```python
from build123d import *

# Parameters (mm, degrees)
F0_W      = 19.05
F0_H      = 19.05
F1_DEPTH  = 11.43
F3_DEPTH  = 19.051
F5_DEPTH  = 19.051
F6_R      = 4.445
F6_R_2    = 1.807104104
F7_DEPTH  = 19.05
F8_DEPTH  = 19.0510001
F9_W      = 2.54
F9_H      = 19.05
F10_DEPTH = 19.0510001
F11_W     = 13.97
F11_H     = 13.97
F11_R     = 4.445
F12_DEPTH = 6.35
F13_R     = 1.27


with BuildPart() as f1:
    # F0 (on Front) → F1 (new body)
    with BuildSketch(Plane.XZ):
        Rectangle(F0_W, F0_H)
    extrude(amount=F1_DEPTH)

    # F2 (on face) → F3 (cut, through all)
    with BuildSketch(Plane.YZ.offset(9.525)):
        with BuildLine():
            Line((0, -9.525), (0, 9.525))
            ThreePointArc((0, 9.525), (-2.032, 0), (0, -9.525))
        make_face()
    extrude(amount=-F3_DEPTH, mode=Mode.SUBTRACT)

    # F4 (on face) → F5 (cut, through all)
    with BuildSketch(Plane.XY.offset(9.525)):
        with BuildLine():
            ThreePointArc((9.525, 0), (19.5841950931, 8.6107735797), (23.34021875, 21.30821875))
            ThreePointArc((23.34021875, 21.30821875), (-12.6974451703, 40.8924138431), (-9.525, 0))
            Line((-9.525, 0), (9.525, 0))
        make_face()
        with BuildLine():
            Line((9.525, 0), (-9.525, 0))
            ThreePointArc((-9.525, 0), (0, -2.032), (9.525, 0))
        make_face()
    extrude(amount=-F5_DEPTH, mode=Mode.SUBTRACT)

    # F6 (on face) → F7 (join)
    with BuildSketch(Plane.XZ.offset(11.43)):
        Circle(F6_R)
        Circle(F6_R_2, mode=Mode.SUBTRACT)
    extrude(amount=-F7_DEPTH)

    # F6 (on face) → F8 (cut, through all)
    with BuildSketch(Plane.XZ.offset(11.43)):
        Circle(F6_R_2)
    extrude(amount=-F8_DEPTH, mode=Mode.SUBTRACT)

    # F9 (on face) → F10 (cut, through all)
    with BuildSketch(Plane.YZ.offset(9.525)):
        with Locations((-10.16, 0)):
            Rectangle(F9_W, F9_H)
    extrude(amount=-F10_DEPTH, mode=Mode.SUBTRACT)

    # F11 (on face) + F6 (on face) → F12 (cut)
    with BuildSketch(Plane.XZ.offset(11.43)):
        Rectangle(F11_W, F11_H)
        Circle(F11_R, mode=Mode.SUBTRACT)
    with BuildSketch(Plane.XZ.offset(11.43)):
        Circle(F6_R)
        Circle(F6_R_2, mode=Mode.SUBTRACT)
    extrude(amount=-F12_DEPTH, mode=Mode.SUBTRACT)

    # F13
    f13_edges = [f1.edges().sort_by_distance(p)[0] for p in [
        (-9.525, -4.445, -9.525),
        (-9.525, -4.445, 9.525),
        (9.525, -4.445, 9.525),
        (9.525, -4.445, -9.525),
    ]]
    fillet(f13_edges, radius=F13_R)


solid = f1.part
```
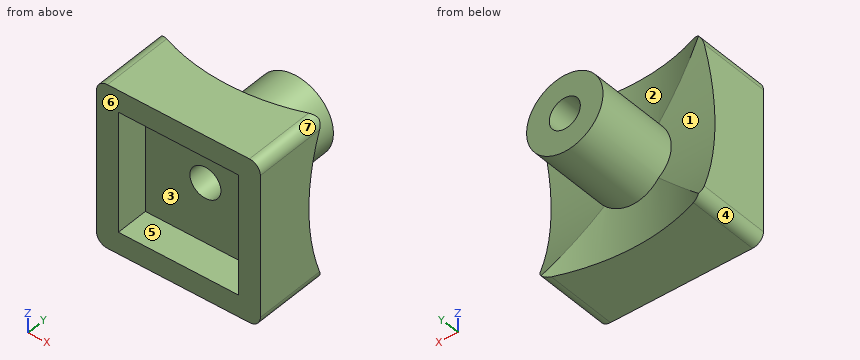
Verification items for the finished model (mm, model axes). Face numbers are marked on the shaded views. A direction names the side the tool comes from. Round coordinates to 2 decimals unless told otherwise and drop trailing zeros. Write each loop counter-clockwise with the first axis right and the second up, starting at its lowest first coordinate (ties: lowest second). Pieces come first, ordered by that corner, then holes.
1. Section check A-A on x = 0. Enter the section's corners in (y, z) (3 decimals), plus the area to 3 significant figures.
2. Gauge pin test, flat ends, axial feed: P1, Ø5, axis at x = 7.5, y = 3.5, coming from the +Z side; P2, Ø7, axis at x = 0.5, z = -3, coming from the -Y side; P3, Ø2, axis at x = -2.5, y = 2, coming from the +Z side; P4, Ø3, axis at x = 2, y = 2.5, coming from the -Z side. Record the tip position at first contact, or that the pin passes through.
3. Section check D-D on x = 5.75. Enter the section's corners in (y, z) (3 decimals), plus the area to 3 significant figures.
4. Scan lines: L1, parallel to X at y = 0.75, z = 0 (3 decimals); L2, parallel to X at y = -3.5, z = 0 (3 decimals). Record each from-to range of solid material in increasing order.
5. Draft check along X on the marked faces 4, 5, 6 and 7. Enter one of: +X half, -X half, draft (parallel to the pull), parting line (faces both ways), or undercut.
6. Section check C-C on z = 0. Enter the section's corners in (x, y) (3 decimals), plus the area to 3 significant figures.
7. Section check B-B on y = -1.25. Enter the section's corners in (x, z) (3 decimals).
8. Access from +Z, -Z, +X, -X, +Y, -Y to the whole of each face (thin tool, end or side, straight path). Record for the marked faces 1, 2 and 3.
Answer:
1. outline: (-8.89, -9.525) - (-2.032, -9.525) - (-2.032, -4.445) - (7.62, -4.445) - (7.62, -1.807) - (-5.08, -1.807) - (-5.08, -6.985) - (-8.89, -6.985) - close; (-8.89, 6.985) - (-5.08, 6.985) - (-5.08, 1.807) - (7.62, 1.807) - (7.62, 4.445) - (-2.032, 4.445) - (-2.032, 9.525) - (-8.89, 9.525) - close
1. area: 117 mm2
2. P1: passes through
2. P2: stops at y = -5.08
2. P3: stops at z = 4.18
2. P4: stops at z = -4.42
3. outline: (-8.89, -9.525) - (-1.313, -9.525) - (-1.313, -5.75) arc R23.34 cw to (-1.313, 5.75) - (-1.313, 9.525) - (-8.89, 9.525) - (-8.89, 6.985) - (-5.08, 6.985) - (-5.08, -6.985) - (-8.89, -6.985) - close
3. area: 85.6 mm2
4. L1: x = -4.445 to -1.807, 1.807 to 4.445
4. L2: x = -9.525 to -1.807, 1.807 to 9.525
5. face 4: -X half
5. face 5: undercut
5. face 6: draft
5. face 7: +X half
6. outline: (-9.525, -8.89) - (-6.985, -8.89) - (-6.985, -5.08) - (-1.807, -5.08) - (-1.807, 7.62) - (-4.445, 7.62) - (-4.445, -2.032) - (-9.525, -2.032) - close; (1.807, -5.08) - (6.985, -5.08) - (6.985, -8.89) - (9.525, -8.89) - (9.525, -2.032) - (4.445, -2.032) - (4.445, 7.62) - (1.807, 7.62) - close
6. area: 117 mm2
7. outline: (-9.525, -8.255) arc R1.27 ccw to (-8.255, -9.525) - (-5.991, -9.525) - (-5.991, -5.991) - (-9.525, -5.991) - close; (-9.525, 5.991) - (-5.991, 5.991) - (-5.991, 9.525) - (-8.255, 9.525) arc R1.27 ccw to (-9.525, 8.255) - close; circle Ø8.89 at (0, 0); (5.991, -9.525) - (8.255, -9.525) arc R1.27 ccw to (9.525, -8.255) - (9.525, -5.991) - (5.991, -5.991) - close; (5.991, 5.991) - (9.525, 5.991) - (9.525, 8.255) arc R1.27 ccw to (8.255, 9.525) - (5.991, 9.525) - close; hole circle Ø3.614 at (0, 0)
8. face 1: -X, +Y
8. face 2: +Z, +Y
8. face 3: -Y
